For this review, take the finished solid that the model builds, in its own axes (mm). A direction names the side the tool comes from. Give positions to 0.01 mm unless a question says otherwise; leave off trailing zeros. Write each loop counter-clockwise with the first axis right and the second up, starting at its lowest first coordinate (ties: lowest second). Pieces come first, ordered by that corner, then holes.
1) For P1, Ø2, axis at x = 26, y = 4.5, coming from the -Z side; P2, Ø11, axis at x = 3.5, y = 8.5, coming from the +Z side; P3, Ø8, axis at y = 3.5, z = 27, coming from the +X side; P4, Ø2, axis at y = 6, z = 23.5, coming from the -X side, all flat-tipped, find the tip position at first contact; note any pin that passes through.
2) We need section B-B on y = 16.25. Give the boundary of the cut face in (x, z).
3) Machinability: for faces 5 (the face through (0, 12, 10)), 6 (the face through (25, 12, 20)), 7 (the face through (5, 12, 20)), which of the approach directions +Z, -Z, +X, -X, +Y, -Y give a long, thin tool a straight path to every point of the face, cutting with its end or side? Answer none if there is none.
4) We need section C-C on y = 3.25. Give the boundary of the cut face in (x, z).
5) Draft analysis for pull direction Z (two halves, no side actions). For faces 1 (the face through (20, 7, 30)), 2 (the face through (15, 13, 35)), 3 (the face through (15, 12, 0)), 4 (the face through (15, 12, 40)), state which applies: pulls with the +Z half, pulls with the -Z half, needs draft (parallel to the pull), parting line crosses it, or undercut.
6) We need section A-A on z = 30. Give the boundary of the cut face in (x, y), and give its area (3 significant figures).
7) Wall thickness on line 1 along Y through (x, z) = (13, 30); line 2 along Z through (x, y) = (16, 13); line 3 along Z through (x, y) = (8.25, 1): over which ranges is each line inside the solid? List them lowest first.
8) We need section D-D on x = 8.75. Give the boundary of the cut face in (y, z).
Autodesk Inventor part; units mm, degrees
ref_plane "YZ Plane" through (0, 0, 0) normal (1, 0, 0) x (0, 1, 0)
ref_plane "XZ Plane" through (0, 0, 0) normal (0, 1, 0) x (-1, 0, 0)
ref_plane "XY Plane" through (0, 0, 0) normal (0, 0, 1) x (1, 0, 0)
sketch "Sketch1" plane through (0, 0, 0) normal (0, 0, 1) x (1, 0, 0)
  line L0 (0, 0) -> (30, 0)
  line L1 (30, 0) -> (30, 23)
  line L2 (30, 23) -> (0, 23)
  line L3 (0, 23) -> (0, 0)
  dimension "d0" = 30
  dimension "d1" = 23
extrude "Extrusion1" add sketch "Sketch1" along normal blind 20
sketch "Sketch2" plane through (0, 0, 20) normal (0, 0, 1) x (1, 0, 0)
  line L0 (30, 23) -> (0, 23)
  line L1 (0, 23) -> (0, 13)
  line L2 (0, 23) -> (0, 0)
  dimension "d4" = 10
sketch "Sketch3" plane through (0, 0, 20) normal (0, 0, 1) x (1, 0, 0)
  point P0 (0, 0)
sketch "Sketch4" plane through (0, 0, 20) normal (0, 0, 1) x (1, 0, 0)
  line L0 (0, 23) -> (0, 0)
  line L1 (0, 13) -> (0, 20)
  dimension "d5" = 7
sketch "Sketch5" plane through (0, 0, 20) normal (0, 0, 1) x (1, 0, 0)
  line L0 (0, 23) -> (0, 0)
  line L1 (0, 13) -> (0, 18)
  dimension "d6" = 5
sketch "Sketch6" plane through (0, 0, 20) normal (0, 0, 1) x (1, 0, 0)
  line L0 (0, 23) -> (10, 23)
  line L1 (30, 23) -> (0, 23)
  line L2 (10, 23) -> (20, 23)
  line L3 (0, 0) -> (30, 0)
  line L4 (10, 23) -> (20, 23)
  line L5 (20, 23) -> (20, 0)
  line L6 (20, 0) -> (10, 0)
  line L7 (10, 0) -> (10, 23)
  dimension "d7" = 10
  dimension "d8" = 10
extrude "Extrusion2" add sketch "Sketch6" along normal blind 20
sketch "Sketch7" plane through (20, 0, 20) normal (1, 0, 0) x (0, 0, -1)
  line L0 (0, 23) -> (-20, 23)
  line L1 (-20, 23) -> (-20, 13)
  line L2 (-20, 23) -> (-20, 0)
  line L3 (-20, 13) -> (-10, 13)
  circle A0 centre (-10, 13) radius 5
  point P0 (20, 0)
  dimension "d11" = 10
  dimension "d12" = 10
  dimension "d13" = 10
extrude "Extrusion3" cut sketch "Sketch7" against normal blind 20
equation "\"BendRadius\" = Thickness"
equation "\"BendReliefWidth\" = Thickness"
equation "\"BendReliefDepth\" = 0.5 * Thickness"
equation "\"CornerReliefSize\" = 4 * Thickness"
equation "\"MinimumRemnant\" = 2 * Thickness"
equation "\"TransitionRadius\" = BendRadius"
equation "\"JacobiRadiusSize\" = BendRadius"
equation "\"GapSize\" = Thickness"
properties part number "pusher"
Results list:
1. P1: stops at z = 0
1. P2: stops at z = 20
1. P3: stops at x = 20
1. P4: stops at x = 10
2. outline: (0, 0) - (30, 0) - (30, 20) - (20, 20) - (20, 26.2) - (10, 26.2) - (10, 20) - (0, 20) - close; (10, 33.8) - (20, 33.8) - (20, 40) - (10, 40) - close
3. face 5: +Z, -Z, -X, +Y, -Y
3. face 6: +Z, +X, +Y, -Y
3. face 7: +Z, -X, +Y, -Y
4. outline: (0, 0) - (30, 0) - (30, 20) - (20, 20) - (20, 40) - (10, 40) - (10, 20) - (0, 20) - close
5. face 1: needs draft
5. face 2: undercut
5. face 3: pulls with the -Z half
5. face 4: pulls with the +Z half
6. outline: (10, 0) - (20, 0) - (20, 8) - (10, 8) - close; (10, 18) - (20, 18) - (20, 23) - (10, 23) - close
6. area: 130 mm2
7. line 1: y = 0 to 8, 18 to 23
7. line 2: z = 0 to 25, 35 to 40
7. line 3: z = 0 to 20
8. outline: (0, 0) - (23, 0) - (23, 20) - (0, 20) - close
